Work out the finished part from the listing and answer in its coordinate system (mm). Face numbers are marked on the shaded views. A direction names the side the tool comes from. Round coordinates to 2 decimals unless told otherwise and drop trailing zeros. Order: outer loops, then holes, each group sorted by start corner. A loop starts at its lowest first (then second) coordinate and runs counter-clockwise, first axis right, second up. Notation, with made-up numbers: (-5.75, 26) -> (15.25, 26) arc R11 ccw to (15.25, 30) -> close; hole circle Ø1 at (86, 37.5). An arc over 180 degrees is marked (long way). Use one line per item in the form item = value.
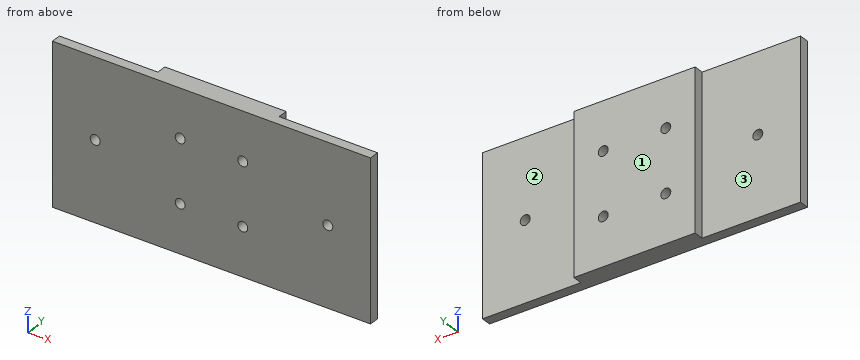
```python
from build123d import *

# Parameters (mm, degrees)
F0_R     = 3.175
F1_DEPTH = 12.7
F2_W     = 62.84501
F2_H     = 6.35
F3_DEPTH = 101.601
F4_DEPTH = 101.601


with BuildPart() as f1:
    # F0 (on Front) → F1 (new body)
    with BuildSketch(Plane.XZ):
        with BuildLine():
            Line((0, 50.8), (-101.6, 50.8))
            Line((-101.6, 50.8), (-101.6, 0))
            Line((-101.6, 0), (-77.47, 0))
            ThreePointArc((-77.47, 0), (-74.295, 3.175), (-71.12, 0))
            Line((-71.12, 0), (0, 0))
            Line((0, 0), (0, 50.8))
        make_face()
        with Locations((-19.99996, 19.99996)):
            Circle(F0_R, mode=Mode.SUBTRACT)
        with BuildLine():
            Line((101.6, 50.8), (0, 50.8))
            Line((0, 50.8), (0, 0))
            Line((0, 0), (71.12, 0))
            ThreePointArc((71.12, 0), (74.295, 3.175), (77.47, 0))
            Line((77.47, 0), (101.6, 0))
            Line((101.6, 0), (101.6, 50.8))
        make_face()
        with Locations((19.97964, 19.99996)):
            Circle(F0_R, mode=Mode.SUBTRACT)
        with BuildLine():
            Line((-77.47, 0), (-101.6, 0))
            Line((-101.6, 0), (-101.6, -50.8))
            Line((-101.6, -50.8), (0, -50.8))
            Line((0, -50.8), (0, 0))
            Line((0, 0), (-71.12, 0))
            ThreePointArc((-71.12, 0), (-74.295, -3.175), (-77.47, 0))
        make_face()
        with Locations((-19.99996, -19.97964)):
            Circle(F0_R, mode=Mode.SUBTRACT)
        with BuildLine():
            Line((71.12, 0), (0, 0))
            Line((0, 0), (0, -50.8))
            Line((0, -50.8), (101.6, -50.8))
            Line((101.6, -50.8), (101.6, 0))
            Line((101.6, 0), (77.47, 0))
            ThreePointArc((77.47, 0), (74.295, -3.175), (71.12, 0))
        make_face()
        with Locations((19.97964, -19.97964)):
            Circle(F0_R, mode=Mode.SUBTRACT)
    extrude(amount=F1_DEPTH)

    # F2 (on face) → F3 (cut, through all)
    with BuildSketch(Plane.XY.offset(50.8)):
        with Locations((-70.177495, -3.175)):
            Rectangle(F2_W, F2_H)
    extrude(amount=-F3_DEPTH, mode=Mode.SUBTRACT)

    # F2 (on face) → F4 (cut, through all)
    with BuildSketch(Plane.XY.offset(50.8)):
        with Locations((70.177495, -3.175)):
            Rectangle(F2_W, F2_H)
    extrude(amount=-F4_DEPTH, mode=Mode.SUBTRACT)


solid = f1.part
```
Item 1: Consider line 1 along X through (y, z) = (-11.5, -20); line 2 along X through (y, z) = (-10, 20.5); line 3 along Y through (x, z) = (-42, 0). Determine where each line is inside the solid, lowest interval first.
Findings:
line_1 = -101.6 to -23.17, -16.83 to 16.8, 23.15 to 101.6
line_2 = -101.6 to -23.14, -16.86 to 16.84, 23.12 to 101.6
line_3 = -12.7 to -6.35
Item 2: The part is cut by section A-A, the plane z = 0. Give the vertices of the cut face in (x, y) (3 decimals).
Findings:
outline = (-101.6, -12.7) -> (-77.47, -12.7) -> (-77.47, -6.35) -> (-101.6, -6.35) -> close; (-71.12, -12.7) -> (71.12, -12.7) -> (71.12, -6.35) -> (38.755, -6.35) -> (38.755, 0) -> (-38.755, 0) -> (-38.755, -6.35) -> (-71.12, -6.35) -> close; (77.47, -12.7) -> (101.6, -12.7) -> (101.6, -6.35) -> (77.47, -6.35) -> close
Item 3: For the marked faces 1, 2 and 3, determine the directions among +Z, -Z, +X, -X, +Y, -Y from which every point of the face is accessible in a straight line to the end or side of a thin tool.
Findings:
face_1 = +Z, -Z, +X, -X, +Y
face_2 = +Z, -Z, +X, +Y
face_3 = +Z, -Z, -X, +Y
Item 4: Flat-ended cylindrical pins translate along their axes: P1, Ø3, axis at y = -2.5, z = 7.5, coming from the -X side (3 decimals); P2, Ø8, axis at x = 56.5, z = -6, coming from the +Y side; P3, Ø5, axis at y = -2, z = -15.5, coming from the +X side (3 decimals); P4, Ø10, axis at x = -20, z = 20, coming from the -Y side. Find the tip coordinate at first contact, or state that the pin passes through.
Findings:
P1 = -38.755
P2 = -6.35
P3 = 38.755
P4 = -12.7
Item 5: The part is cut by section B-B, the plane x = -87. Give the vertices of the cut face in (y, z), and give its area (3 significant figures).
Findings:
outline = (-12.7, -50.8) -> (-6.35, -50.8) -> (-6.35, 50.8) -> (-12.7, 50.8) -> close
area = 645 mm^2
